Geometry: final body of the model. Coordinates: model frame, mm. Face numbers are marked on the shaded views. Give positions to 0.01 mm unless a question says otherwise; leave off trailing zeros. Loops run counter-clockwise (first coordinate to the right, second up) from the corner with the lowest first, then second, coordinate; pieces in that order, holes last. Notation, with made-up numbers: (28.25, 30.5) - (76.25, 30.5) arc R33 ccw to (76.25, 64.5) - close; hole circle Ø9 at (37.25, 55). An arc over 180 degrees is marked (long way). Use one line per item in the form item = value.
```python
from build123d import *

# Parameters (mm, degrees)
EXTRUDE_1_DEPTH     = 1.2
SKETCH_2_R          = 1.6
CUT_EXTRUDE_1_DEPTH = 1.2
SKETCH_4_W          = 20
SKETCH_4_H          = 1.2


with BuildPart() as part:
    # 草图1 → 凸台-拉伸1 (new body)
    with BuildSketch(Plane.XY):
        with BuildLine():
            Line((7.478060046, -4.57852194), (10.978060046, -4.57852194))
            ThreePointArc((10.978060046, -4.57852194), (15.220700733, -2.821162627), (16.978060046, 1.42147806))
            Line((16.978060046, 1.42147806), (16.978060046, 2.42147806))
            ThreePointArc((16.978060046, 2.42147806), (15.220700733, 6.664118747), (10.978060046, 8.42147806))
            Line((10.978060046, 8.42147806), (-16.021939954, 8.42147806))
            ThreePointArc((-16.021939954, 8.42147806), (-20.264580641, 6.664118747), (-22.021939954, 2.42147806))
            Line((-22.021939954, 2.42147806), (-22.021939954, 1.42147806))
            ThreePointArc((-22.021939954, 1.42147806), (-20.264580641, -2.821162627), (-16.021939954, -4.57852194))
            Line((-16.021939954, -4.57852194), (-12.521939954, -4.57852194))
            Line((-12.521939954, -4.57852194), (-12.521939954, -7.57852194))
            Line((-12.521939954, -7.57852194), (7.478060046, -7.57852194))
            Line((7.478060046, -7.57852194), (7.478060046, -4.57852194))
        make_face()
    extrude(amount=EXTRUDE_1_DEPTH)

    # 草图2 → 切除-拉伸1 (cut)
    with BuildSketch(Plane.XY.offset(1.2)):
        with Locations((-14.521939954, 1.92147806)):
            Circle(SKETCH_2_R)
        with Locations((9.478060046, 1.92147806)):
            Circle(SKETCH_2_R)
    extrude(amount=-CUT_EXTRUDE_1_DEPTH, mode=Mode.SUBTRACT)

    # 扫描1: sweep along a path in 草图3
    with BuildLine(Plane.ZY.offset(12.521939954)) as sweep_1_path:
        ThreePointArc((0.6, -7.57852194), (2.762027547, -9.176177297), (4.561146836, -7.178669966))
    # 草图4 → 扫描1 (sweep)
    with BuildSketch(Plane.XZ.offset(7.57852194)):
        with Locations((-2.521939954, 0.6)):
            Rectangle(SKETCH_4_W, SKETCH_4_H)
    sweep(path=sweep_1_path.line)


solid = part.part
```
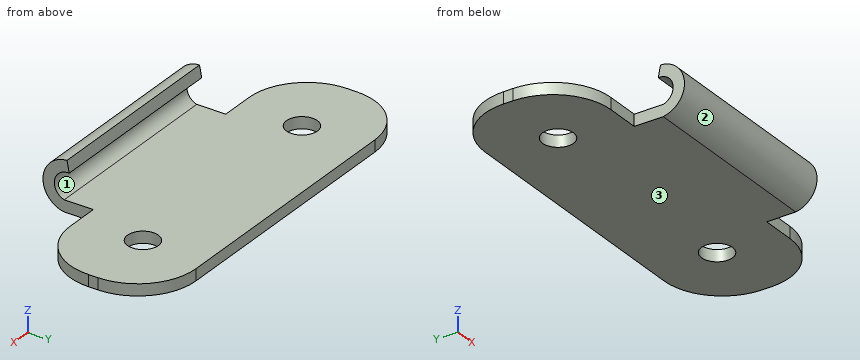
(1) Cut plane D-D (y = 3). Return the cut outline in (x, z), plus the area to 3 significant figures.
Solution:
outline = (-21.99, 0) - (-15.7, 0) - (-15.7, 1.2) - (-21.99, 1.2) - close; (-13.34, 0) - (8.3, 0) - (8.3, 1.2) - (-13.34, 1.2) - close; (10.66, 0) - (16.95, 0) - (16.95, 1.2) - (10.66, 1.2) - close
area = 41.1 mm2
(2) Pull-direction query (Z, two-part tool) for the marked faces 1, 2 and 3; classes: released by +Z, released by -Z, zero draft, split by the parting line, or undercut.
Solution:
face_1 = undercut
face_2 = split by the parting line
face_3 = released by -Z
(3) Cut plane A-A (y = -8.25). Return the cut outline in (x, z).
Solution:
outline = (-12.52, 0.2) - (7.48, 0.2) - (7.48, 1.63) - (-12.52, 1.63) - close; (-12.52, 3.5) - (7.48, 3.5) - (7.48, 4.92) - (-12.52, 4.92) - close
(4) Material intervals for L1, parallel to X at y = -9, z = 3.15; L2, parallel to Z at x = -18, y = 4.75; L3, parallel to Y at x = -8.5, z = 4.95, sorted ascending. Write a range as from..to.
Solution:
L1 = -12.52..7.48
L2 = 0..1.2
L3 = -8.19..-7.25
(5) Cut plane B-B (x = -5.5). Return the cut outline in (y, z), plus the area to 3 significant figures.
Solution:
outline = (-7.58, 0) - (8.42, 0) - (8.42, 1.2) - (-7.58, 1.2) arc R1.42 cw to (-7.06, 3.97) - (-7.29, 5.15) arc R2.59 ccw to start
area = 26.1 mm2
(6) Cut plane C-C (z = 0.4). Return the cut outline in (x, y), plus the area to 3 significant figures.
Solution:
outline = (-22.02, 1.42) arc R6 ccw to (-16.02, -4.58) - (-12.52, -4.58) - (-12.52, -8.62) - (7.48, -8.62) - (7.48, -4.58) - (10.98, -4.58) arc R6 ccw to (16.98, 1.42) - (16.98, 2.42) arc R6 ccw to (10.98, 8.42) - (-16.02, 8.42) arc R6 ccw to (-22.02, 2.42) - close; hole circle Ø3.2 at (-14.52, 1.92); hole circle Ø3.2 at (9.48, 1.92)
area = 541 mm2
(7) Pin query (flat end, axial travel): P1, Ø1, axis at x = -15, z = 0.5, coming from the -Y side; P2, Ø8, axis at x = 11, y = -3, coming from the +Z side; P3, Ø3, axis at x = 9.48, y = 1.92, coming from the -Z side; P4, Ø2.5, axis at y = -8, z = 2, coming from the -X side. Return the tip coordinate at first contact, or that it passes through.
Solution:
P1 = -4.58
P2 = 1.2
P3 = through
P4 = -12.52
